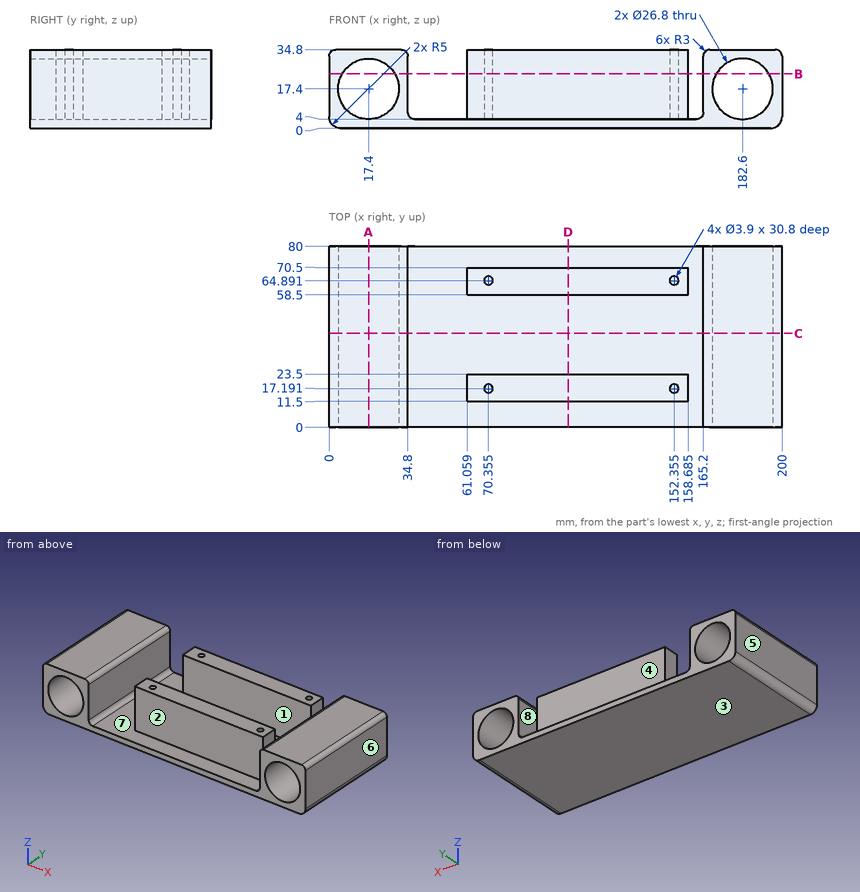
For this review, use the dimensioned drawing (mm, ordinates from the lowest corner) and the shaded views. A direction names the side the tool comes from. Round coordinates to 2 decimals unless told otherwise and drop trailing zeros. Order: outer loops, then holes, each group sorted by start corner. A loop starts at its lowest first (then second) coordinate and runs counter-clockwise, first axis right, second up. Notation, with made-up numbers: (59, -20.5) -> (111, -20.5) arc R23 ccw to (111, 7.5) -> close; hole circle Ø6 at (32, -2). An arc over 180 degrees is marked (long way). Use CSV: the item, a comma, the result in double quotes. Start each with the question number.
(1) Insertion check: pin 1 (4.5 mm diameter, centred on x = 70.36, y = 64.89, fed in from -Z); pin 2 (1.2 mm diameter, centred on x = 152.5, y = 18, fed in from +Z); pin 3 (4 mm diameter, centred on x = 145.5, z = 7, fed in from -Y); pin 4 (15.5 mm diameter, centred on x = 110.5, z = 24.5, fed in from +Y). Each pin has a flat end and moves straight along its axis. Give the tip position at first contact, or say it passes through.
(2) Tool access review of the marked faces 4, 5, 6, 7 and 8: name each direction out of +Z, -Z, +X, -X, +Y, -Y from which nothing blocks a thin tool from reaching the whole face with its end or side.
(3) Mouldability with a two-part tool opening along Y and no side actions: class the marked faces 1, 2 and 3 as pulls with the +Y half, pulls with the -Y half, needs draft (parallel to the pull), parting line crosses it, or undercut.
(4) Wall thickness on probe 1 along X at (y, z) = (47, 17) (1 decimal); probe 2 along X at (y, z) = (59, 17) (1 decimal); probe 3 along Y at (x, z) = (100, 5.5): over which ranges is each line inside the solid? List them lowest first. Write a range as from..to.
(5) Consider section C-C on y = 41.5. Write out the cut boundary in (x, z).
(6) Consider section D-D on x = 105.5. Write out the cut boundary in (y, z).
(7) Consider section A-A on x = 17.4. Write out the cut boundary in (y, z), and give its area (3 significant figures).
(8) Consider section B-B on z = 24. State how many separate pieces and enclosed holes the cut face has, and give its area (3 significant figures).
Responses:
1,pin 1,"z = 0"
1,pin 2,"z = 4"
1,pin 3,"y = 11.5"
1,pin 4,"y = 70.5"
2,face 4,"+Z, +Y"
2,face 5,"+Z, -Z, -X, +Y, -Y"
2,face 6,"+Z, -Z, +X, +Y, -Y"
2,face 7,"+Z"
2,face 8,"+Z, +Y, -Y"
3,face 1,"undercut"
3,face 2,"pulls with the -Y half"
3,face 3,"needs draft"
4,probe 1,"0..4, 30.8..34.8, 165.2..169.2, 196..200"
4,probe 2,"0..4, 30.8..34.8, 61.1..158.7, 165.2..169.2, 196..200"
4,probe 3,"11.5..23.5, 58.5..70.5"
5,outline,"(0, 5) arc R5 ccw to (5, 0) -> (195, 0) arc R5 ccw to (200, 5) -> (200, 31.8) arc R3 ccw to (197, 34.8) -> (168.2, 34.8) arc R3 ccw to (165.2, 31.8) -> (165.2, 7) arc R3 cw to (162.2, 4) -> (37.8, 4) arc R3 cw to (34.8, 7) -> (34.8, 31.8) arc R3 ccw to (31.8, 34.8) -> (3, 34.8) arc R3 ccw to (0, 31.8) -> close; hole circle Ø26.8 at (17.4, 17.4); hole circle Ø26.8 at (182.6, 17.4)"
6,outline,"(0, 0) -> (80, 0) -> (80, 4) -> (70.5, 4) -> (70.5, 34.8) -> (58.5, 34.8) -> (58.5, 4) -> (23.5, 4) -> (23.5, 34.8) -> (11.5, 34.8) -> (11.5, 4) -> (0, 4) -> close"
7,outline,"(0, 0) -> (80, 0) -> (80, 4) -> (0, 4) -> close; (0, 30.8) -> (80, 30.8) -> (80, 34.8) -> (0, 34.8) -> close"
7,area,"640 mm²"
8,separate pieces,"6"
8,enclosed holes,"4"
8,area,"4,130 mm²"
